Can you work these out from the model? Positions are in its coordinate system, mm. Round coordinates to 2 decimals unless told otherwise and drop trailing zeros. Loops run counter-clockwise (first coordinate to the right, second up) from the corner with the lowest first, then second, coordinate; pieces in that order, holes last.
(1) I want a section at C-C on z = 1.75. Give the number of separate pieces and of enclosed holes in the cut face, plus the area to 3 significant figures.
(2) I want a section at A-A on x = -67. Write out the boundary of the cut face in (y, z), plus the area to 3 significant figures.
(3) I want a section at B-B on y = 0. Write out the boundary of the cut face in (x, z), plus the area to 3 significant figures.
(4) I want a section at D-D on x = -20. Write out the boundary of the cut face in (y, z).
(5) Will these pins go through, and if not, where does the flat tip stop? pin 1 Ø5 at (x, y) = (-15.25, 15.25) entering from -Z; pin 2 Ø1 at (x, z) = (-36.5, 1.5) entering from +Y.
(6) If I drill on line 1 along Y through (x, z) = (8, 2.2); line 2 along Y through (x, z) = (-24, 0.3); line 3 along X through (y, z) = (16.5, 1.05), over which ranges is the centre line in solid material (lowest first)?
from build123d import *

# Parameters (mm, degrees)
CROQUIS1_R              = 2.25
CROQUIS1_R_2            = 3
CROQUIS1_R_3            = 1.5
CROQUIS1_R_4            = 2.249997567
SALIENTE_EXTRUIR1_DEPTH = 2.5
SALIENTE_EXTRUIR3_START = -2.5
CROQUIS6_R              = 2.250000066
CROQUIS6_R_2            = 1.5
CROQUIS6_R_3            = 2.25
SALIENTE_EXTRUIR3_DEPTH = 2.5
CROQUIS5_R              = 22.5
CROQUIS5_R_2            = 1
CROQUIS5_R_3            = 2
CORTAR_EXTRUIR5_DEPTH   = 2.5
CORTAR_EXTRUIR6_DEPTH   = 2.5
REDONDEO1_R             = 2
CROQUIS11_R             = 1.5
CROQUIS11_R_2           = 1.500000006
CORTAR_EXTRUIR7_DEPTH   = 2.5


with BuildPart() as part:
    # Croquis1 → Saliente-Extruir1 (new body)
    with BuildSketch(Plane.XY):
        with BuildLine():
            Line((-29.502526327, -44.949972179), (-23.17778065, -37.243838032))
            ThreePointArc((-23.17778065, -37.243838032), (-18.839723212, -32.444384768), (-14.046056443, -28.099933953))
            ThreePointArc((-14.046056443, -28.099933953), (-12.991422185, -27.658257217), (-11.867164621, -27.866527921))
            ThreePointArc((-11.867164621, -27.866527921), (-11.203313373, -28.112469078), (-10.500314, -28.196))
            Line((-10.500314, -28.196), (10.499686, -28.196))
            ThreePointArc((10.499686, -28.196), (11.203007921, -28.112542722), (11.867164264, -27.866528101))
            ThreePointArc((11.867164264, -27.866528101), (12.991422421, -27.658256674), (14.046057406, -28.099933523))
            ThreePointArc((14.046057406, -28.099933523), (18.839775902, -32.444337151), (23.177889012, -37.243749049))
            Line((23.177889012, -37.243749049), (29.502526012, -44.949972049))
            ThreePointArc((29.502526012, -44.949972049), (40.113877497, -46.255199126), (41.931739547, -35.719556022))
            Line((41.931739547, -35.719556022), (21.72923101, -5.566101046))
            ThreePointArc((21.72923101, -5.566101046), (20.036969431, -9.5e-08), (21.729230693, 5.566100954))
            Line((21.729230693, 5.566100954), (41.931739693, 35.719555954))
            ThreePointArc((41.931739693, 35.719555954), (40.113877277, 46.255198335), (29.502526336, 44.949972165))
            Line((29.502526336, 44.949972165), (23.17778065, 37.243838007))
            ThreePointArc((23.17778065, 37.243838007), (18.839723212, 32.444384742), (14.046056443, 28.099933927))
            ThreePointArc((14.046056443, 28.099933927), (12.991421988, 27.658257139), (11.867164252, 27.866528027))
            ThreePointArc((11.867164252, 27.866528027), (11.203313175, 28.112469073), (10.500314, 28.195999974))
            Line((10.500314, 28.195999974), (-10.500314, 28.195999974))
            ThreePointArc((-10.500314, 28.195999974), (-11.203313178, 28.112469098), (-11.867164264, 27.866528075))
            ThreePointArc((-11.867164264, 27.866528075), (-12.991422421, 27.658256648), (-14.046057406, 28.099933497))
            ThreePointArc((-14.046057406, 28.099933497), (-18.839775902, 32.444337126), (-23.177889012, 37.243749023))
            Line((-23.177889012, 37.243749023), (-29.502526012, 44.949972023))
            ThreePointArc((-29.502526012, 44.949972023), (-40.146302424, 46.230987494), (-41.886340556, 35.652554517))
            ThreePointArc((-41.886340556, 35.652554517), (-41.288874902, 25.337679941), (-50.13550001, 20.000000021))
            Line((-50.13550001, 20.000000021), (-97.31807601, 20.000000021))
            ThreePointArc((-97.31807601, 20.000000021), (-99.1994919, 19.554558541), (-100.681450855, 18.312809163))
            add(Edge.make_bspline(
                [(-107.31807554, 2.1e-08), (-107.252414123, 7.059743944), (-104.975710329, 13.164639039), (-100.681450855, 18.312809163)],
                knots=[0, 0, 0, 0, 1, 1, 1, 1], degree=3))
            add(Edge.make_bspline(
                [(-107.31807554, 2.1e-08), (-107.252414123, -7.059743902), (-104.975710329, -13.164638997), (-100.681450855, -18.312809121)],
                knots=[0, 0, 0, 0, 1, 1, 1, 1], degree=3))
            ThreePointArc((-100.681450855, -18.312809121), (-99.19949186, -19.554558345), (-97.31807601, -19.9999997))
            Line((-97.31807601, -19.9999997), (-50.13550001, -19.9999997))
            ThreePointArc((-50.13550001, -19.9999997), (-41.288874902, -25.33767962), (-41.886340556, -35.652554196))
            ThreePointArc((-41.886340556, -35.652554196), (-40.146302646, -46.230987042), (-29.502526327, -44.949972179))
        make_face()
        with Locations((-25.371621, 27.641642)):
            Circle(CROQUIS1_R, mode=Mode.SUBTRACT)
        with Locations((-35.493242035, 40.033284004)):
            Circle(CROQUIS1_R, mode=Mode.SUBTRACT)
        with Locations((-35.49324201, -40.0332837)):
            Circle(CROQUIS1_R, mode=Mode.SUBTRACT)
        with Locations((15.25, -15.25)):
            Circle(CROQUIS1_R_2, mode=Mode.SUBTRACT)
        with Locations((35.493242035, -40.03328403)):
            Circle(CROQUIS1_R, mode=Mode.SUBTRACT)
        with Locations((-15.25, 15.25)):
            Circle(CROQUIS1_R_2, mode=Mode.SUBTRACT)
        with Locations((-25.371621, -27.641642)):
            Circle(CROQUIS1_R, mode=Mode.SUBTRACT)
        with Locations((-35.318076, 15.5)):
            Circle(CROQUIS1_R_3, mode=Mode.SUBTRACT)
        with Locations((25.371621, -27.641642)):
            Circle(CROQUIS1_R, mode=Mode.SUBTRACT)
        with Locations((-15.25, -15.25)):
            Circle(CROQUIS1_R_2, mode=Mode.SUBTRACT)
        with Locations((-97.318076, 15.5)):
            Circle(CROQUIS1_R_3, mode=Mode.SUBTRACT)
        with Locations((15.25, 15.25)):
            Circle(CROQUIS1_R_2, mode=Mode.SUBTRACT)
        with Locations((-35.318076, -15.5)):
            Circle(CROQUIS1_R_3, mode=Mode.SUBTRACT)
        with Locations((25.371621, 27.641642)):
            Circle(CROQUIS1_R, mode=Mode.SUBTRACT)
        with Locations((-97.318076, -15.5)):
            Circle(CROQUIS1_R_3, mode=Mode.SUBTRACT)
        with Locations((35.493241695, 40.03328329)):
            Circle(CROQUIS1_R_4, mode=Mode.SUBTRACT)
        with BuildLine():
            Line((10.499686, -24.196), (-10.500314, -24.196))
            ThreePointArc((-10.500314, -24.196), (-11.500314, -25.196), (-10.500314, -26.196))
            Line((-10.500314, -26.196), (10.499686, -26.196))
            ThreePointArc((10.499686, -26.196), (11.499686, -25.196), (10.499686, -24.196))
        make_face(mode=Mode.SUBTRACT)
        with BuildLine():
            Line((10.499686, 24.196), (-10.500314, 24.196))
            ThreePointArc((-10.500314, 24.196), (-11.500314, 25.196), (-10.500314, 26.196))
            Line((-10.500314, 26.196), (10.499686, 26.196))
            ThreePointArc((10.499686, 26.196), (11.499686, 25.196), (10.499686, 24.196))
        make_face(mode=Mode.SUBTRACT)
    extrude(amount=SALIENTE_EXTRUIR1_DEPTH)


with BuildPart() as saliente_extruir3_tool:
    # Croquis6 → Saliente-Extruir3 (new body)
    # profile 1 of 10: a face of its own
    with BuildSketch(Plane.XY.offset(2.5).offset(SALIENTE_EXTRUIR3_START)):
        with Locations((-35.493242163, 40.033284025)):
            Circle(CROQUIS6_R)
        with Locations((-35.493242163, 40.033284025)):
            Circle(CROQUIS6_R_2, mode=Mode.SUBTRACT)
    # profile 2 of 10: a face of its own
    with BuildSketch(Plane.XY.offset(2.5).offset(SALIENTE_EXTRUIR3_START)):
        with Locations((-25.371621, 27.641642)):
            Circle(CROQUIS6_R_3)
        with Locations((-25.371621, 27.641642)):
            Circle(CROQUIS6_R_2, mode=Mode.SUBTRACT)
    # profile 3 of 10: a face of its own
    with BuildSketch(Plane.XY.offset(2.5).offset(SALIENTE_EXTRUIR3_START)):
        with Locations((25.371621, 27.641642)):
            Circle(CROQUIS6_R_3)
        with Locations(Location((25.371621, 27.641642, 0), (0, 0, 180))):
            Circle(CROQUIS6_R_2, mode=Mode.SUBTRACT)
    # profile 4 of 10: a face of its own
    with BuildSketch(Plane.XY.offset(2.5).offset(SALIENTE_EXTRUIR3_START)):
        with Locations((35.493242163, 40.033284025)):
            Circle(CROQUIS6_R)
        with Locations(Location((35.493242163, 40.033284025, 0), (0, 0, 180))):
            Circle(CROQUIS6_R_2, mode=Mode.SUBTRACT)
    # profile 5 of 10: a face of its own
    with BuildSketch(Plane.XY.offset(2.5).offset(SALIENTE_EXTRUIR3_START)):
        with Locations((35.493242163, -40.033284025)):
            Circle(CROQUIS6_R)
        with Locations((35.493242163, -40.033284025)):
            Circle(CROQUIS6_R_2, mode=Mode.SUBTRACT)
    # profile 6 of 10: a face of its own
    with BuildSketch(Plane.XY.offset(2.5).offset(SALIENTE_EXTRUIR3_START)):
        with Locations((25.371621, -27.641642)):
            Circle(CROQUIS6_R_3)
        with Locations((25.371621, -27.641642)):
            Circle(CROQUIS6_R_2, mode=Mode.SUBTRACT)
    # profile 7 of 10: a face of its own
    with BuildSketch(Plane.XY.offset(2.5).offset(SALIENTE_EXTRUIR3_START)):
        with Locations((-25.371621, -27.641642)):
            Circle(CROQUIS6_R_3)
        with Locations(Location((-25.371621, -27.641642, 0), (0, 0, 180))):
            Circle(CROQUIS6_R_2, mode=Mode.SUBTRACT)
    # profile 8 of 10: a face of its own
    with BuildSketch(Plane.XY.offset(2.5).offset(SALIENTE_EXTRUIR3_START)):
        with Locations((-35.493242163, -40.033284025)):
            Circle(CROQUIS6_R)
        with Locations(Location((-35.493242163, -40.033284025, 0), (0, 0, 180))):
            Circle(CROQUIS6_R_2, mode=Mode.SUBTRACT)
    # profile 9 of 10: a face of its own
    with BuildSketch(Plane.XY.offset(2.5).offset(SALIENTE_EXTRUIR3_START)):
        with BuildLine():
            Line((-99.1994919, 19.554558541), (-40.146302424, 46.230987494))
            ThreePointArc((-40.146302424, 46.230987494), (-43.140478024, 41.291171845), (-41.886340556, 35.652554517))
            ThreePointArc((-41.886340556, 35.652554517), (-41.288875033, 25.33768001), (-50.13550001, 20.000000021))
            Line((-50.13550001, 20.000000021), (-97.31807601, 20.000000021))
            ThreePointArc((-97.31807601, 20.000000021), (-98.214581153, 19.590579436), (-99.1994919, 19.554558541))
        make_face()
    # profile 10 of 10: a face of its own
    with BuildSketch(Plane.XY.offset(2.5).offset(SALIENTE_EXTRUIR3_START)):
        with BuildLine():
            Line((-50.13550001, -20.000000021), (-97.31807601, -20.000000021))
            ThreePointArc((-97.31807601, -20.000000021), (-98.214581153, -19.590579436), (-99.1994919, -19.554558541))
            Line((-99.1994919, -19.554558541), (-40.146302424, -46.230987494))
            ThreePointArc((-40.146302424, -46.230987494), (-43.140478024, -41.291171845), (-41.886340556, -35.652554517))
            ThreePointArc((-41.886340556, -35.652554517), (-41.288875033, -25.33768001), (-50.13550001, -20.000000021))
        make_face()
    extrude(amount=SALIENTE_EXTRUIR3_DEPTH)


with BuildPart() as part_1:
    add(part.part)


with BuildPart() as part_2:
    # Saliente-Extruir3: joined with saliente_extruir3_tool
    add(part_1.part.fuse(saliente_extruir3_tool.part, tol=0.00001))

    # Croquis5 → Cortar-Extruir5 (cut)
    with BuildSketch(Plane.XY.offset(2.5)):
        with Locations((-69.81807554, 2.1e-08)):
            Circle(CROQUIS5_R)
        with Locations((-78.402781137, 23.586284803)):
            Circle(CROQUIS5_R_2)
        with Locations((-94.91807554, 2.1e-08)):
            Circle(CROQUIS5_R_2)
        with Locations(Location((-78.402781137, -23.586284761, 0), (0, 0, 180))):
            Circle(CROQUIS5_R_2)
        with Locations((-50.726192448, 19.091883113)):
            Circle(CROQUIS5_R_3)
        with Locations(Location((-50.726192448, -19.091883071, 0), (0, 0, 180))):
            Circle(CROQUIS5_R_3)
    extrude(amount=-CORTAR_EXTRUIR5_DEPTH, mode=Mode.SUBTRACT)

    # Croquis10 → Cortar-Extruir6 (cut)
    with BuildSketch(Plane.XY.offset(2.5)):
        with BuildLine():
            Line((-81.857336743, 19.008055936), (-85.001521285, 25.96828755))
            ThreePointArc((-85.001521285, 25.96828755), (-102.968648752, 18.835514529), (-107.31807554, 2.1e-08))
            ThreePointArc((-107.31807554, 2.1e-08), (-102.968648773, -18.835514521), (-85.001521285, -25.96828755))
            Line((-85.001521285, -25.96828755), (-81.857336743, -19.008055936))
            ThreePointArc((-81.857336743, -19.008055936), (-92.318075557, 0), (-81.857336743, 19.008055936))
        make_face()
    extrude(amount=-CORTAR_EXTRUIR6_DEPTH, mode=Mode.SUBTRACT)

    # Redondeo1
    redondeo1_edges = [part_2.edges().sort_by_distance(p)[0] for p in [
        (-81.857336743, -19.008055936, 1.25),
        (-85.001521285, -25.96828755, 1.25),
        (-85.001521285, 25.96828755, 1.25),
        (-81.857336743, 19.008055936, 1.25),
    ]]
    fillet(redondeo1_edges, radius=REDONDEO1_R)

    # Croquis11 → Cortar-Extruir7 (cut)
    with BuildSketch(Plane.XY.offset(2.5)):
        with Locations((-60.881562628, 32.984594162)):
            Circle(CROQUIS11_R)
        with Locations((-60.881562628, -32.984594162)):
            Circle(CROQUIS11_R_2)
    extrude(amount=-CORTAR_EXTRUIR7_DEPTH, mode=Mode.SUBTRACT)


solid = part_2.part
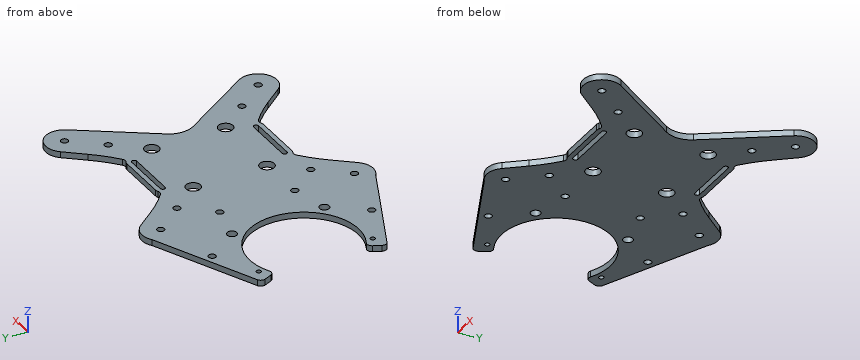
Filled sheet:
1. separate pieces: 1
1. enclosed holes: 22
1. area: 6,600 mm2
2. outline: (-34.1, 0) - (-22.32, 0) - (-22.32, 2.5) - (-34.1, 2.5) - close; (22.32, 0) - (34.1, 0) - (34.1, 2.5) - (22.32, 2.5) - close
2. area: 58.9 mm2
3. outline: (-47.32, 0) - (20.04, 0) - (20.04, 2.5) - (-47.32, 2.5) - close
3. area: 168 mm2
4. outline: (-33.64, 0) - (33.64, 0) - (33.64, 2.5) - (-33.64, 2.5) - close
5. pin 1: passes through
5. pin 2: stops at y = 47.77
6. line 1: y = -28.2 to -26.2, -24.2 to 24.2, 26.2 to 28.2
6. line 2: y = -38.25 to -28.25, -27.03 to 27.03, 28.25 to 38.25
6. line 3: x = -54.52 to -36.44, -34.2 to -17.98, -12.52 to 12.52, 17.98 to 29.05
